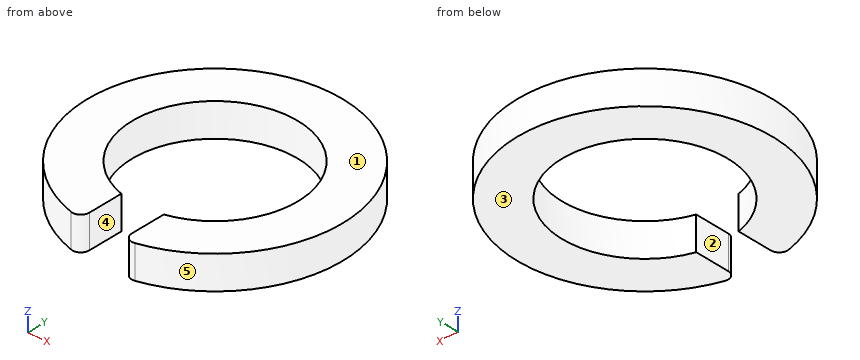
```python
from build123d import *

# Parameters (mm, degrees)
SKETCH1_R           = 7.5
SKETCH1_R_2         = 4.865
BOSS_EXTRUDE1_DEPTH = 1.95
SKETCH2_W           = 2.5
SKETCH2_H           = 4.968115063
CUT_EXTRUDE1_DEPTH  = 11.784363681
FILLET1_R           = 0.5


with BuildPart() as part:
    # Sketch1 → Boss-Extrude1 (new body)
    with BuildSketch(Plane.XY):
        Circle(SKETCH1_R)
        Circle(SKETCH1_R_2, mode=Mode.SUBTRACT)
    extrude(amount=BOSS_EXTRUDE1_DEPTH)

    # Sketch2 → Cut-Extrude1 (cut, through all)
    with BuildSketch(Plane.XY.offset(1.95)):
        with Locations((0, -6.251822647)):
            Rectangle(SKETCH2_W, SKETCH2_H)
    extrude(amount=-CUT_EXTRUDE1_DEPTH, mode=Mode.SUBTRACT)

    # Fillet1
    fillet1_edges = [part.edges().sort_by_distance(p)[0] for p in [
        (-1.25, -7.395099729, 0.975),
        (1.25, -7.395099729, 0.975),
    ]]
    fillet(fillet1_edges, radius=FILLET1_R)


solid = part.part
```
Design review of the part built by this model. Coordinates are the model's own, in mm. Face numbers are marked on the shaded views. A direction names the side the tool comes from. Coordinates: 2 decimals unless noted, no trailing zeros. Loops run counter-clockwise (first coordinate to the right, second up) from the corner with the lowest first, then second, coordinate; pieces in that order, holes last. Notation, with made-up numbers: (40.25, -13.75) - (74.25, -13.75) arc R10 cw to (74.25, -9.75) - close; hole circle Ø5 at (72.5, -24.75). An arc over 180 degrees is marked (long way). Use CSV: the item, a comma, the result in double quotes. Start each with the question number.
1) Consider section B-B on x = 3. Write out the cut boundary in (y, z).
2) For pin 1 Ø1.5 at (x, y) = (-2.5, -1) entering from +Z, flat-tipped, find the tip position at first contact; note if it passes through.
3) Consider section D-D on x = 0. Write out the cut boundary in (y, z) (3 decimals), then the cut area to 3 significant figures.
4) The part is to be moulded in two halves that separate along X. For the marked faces 3, 4 and 5, say which applies: +X half, -X half, draft (parallel to the pull), parting line (faces both ways), or undercut.
5) Tool access review of the marked faces 1 and 2: name each direction out of +Z, -Z, +X, -X, +Y, -Y from which nothing blocks a thin tool from reaching the whole face with its end or side.
6) Consider section A-A on y = 0. Write out the cut boundary in (x, z) (3 decimals).
7) Consider section C-C on z = 1.7. Write out the cut boundary in (x, y) (3 decimals), then the cut area to 3 significant figures.
8) Wall thickness on L1, parallel to X at y = 0, z = 0.8 (3 decimals); L2, parallel to Y at x = 0, z = 1.4 (3 decimals); L3, parallel to X at y = 2.5, z = 0.8: over which ranges is each line inside the solid? List them lowest first. Write a range as from..to.
Geometry says:
1,outline,"(-6.87, 0) - (-3.83, 0) - (-3.83, 1.95) - (-6.87, 1.95) - close; (3.83, 0) - (6.87, 0) - (6.87, 1.95) - (3.83, 1.95) - close"
2,pin 1,"through"
3,outline,"(4.865, 0) - (7.5, 0) - (7.5, 1.95) - (4.865, 1.95) - close"
3,area,"5.14 mm^2"
4,face 3,"draft"
4,face 4,"undercut"
4,face 5,"parting line"
5,face 1,"+Z, +X, -X, +Y, -Y"
5,face 2,"+Z, -Z, -Y"
6,outline,"(-7.5, 0) - (-4.865, 0) - (-4.865, 1.95) - (-7.5, 1.95) - close; (4.865, 0) - (7.5, 0) - (7.5, 1.95) - (4.865, 1.95) - close"
7,outline,"(-1.875, -7.262) arc R0.5 ccw to (-1.25, -6.778) - (-1.25, -4.702) arc R4.865 cw (long way) to (1.25, -4.702) - (1.25, -6.778) arc R0.5 ccw to (1.875, -7.262) arc R7.5 ccw (long way) to start"
7,area,"95.5 mm^2"
8,L1,"-7.5..-4.865, 4.865..7.5"
8,L2,"4.865..7.5"
8,L3,"-7.07..-4.17, 4.17..7.07"
